Source: CAD feature listing. Evaluate the final solid. Frame: model axes, mm. A direction names the side the tool comes from. Give positions to 0.01 mm unless a question says otherwise; leave off trailing zeros. Loops run counter-clockwise (first coordinate to the right, second up) from the corner with the lowest first, then second, coordinate; pieces in that order, holes last. Notation, with made-up numbers: (57.25, -35) -> (67.25, -35) arc R19 cw to (67.25, -19) -> close; hole circle Ø10 at (-11, 67.25). An arc over 180 degrees is marked (long way). Return JSON: item names as keys, results as strings. Group by question number.
```python
from build123d import *

# Parameters (mm, degrees)
SKETCH1_W           = 24.4
SKETCH1_H           = 14
SKETCH1_R           = 1.3
BOSS_EXTRUDE1_DEPTH = 2.6
SKETCH2_W           = 24.4
SKETCH2_H           = 5
BOSS_EXTRUDE2_DEPTH = 11
SKETCH3_R           = 1.6
CUT_EXTRUDE1_DEPTH  = 4.6


with BuildPart() as part:
    # Sketch1 → Boss-Extrude1 (new body)
    with BuildSketch(Plane.XY):
        with Locations((0, 7)):
            Rectangle(SKETCH1_W, SKETCH1_H)
        with Locations((-8.89, 10.6)):
            Circle(SKETCH1_R, mode=Mode.SUBTRACT)
        with Locations((8.89, 10.6)):
            Circle(SKETCH1_R, mode=Mode.SUBTRACT)
    extrude(amount=BOSS_EXTRUDE1_DEPTH)

    # Sketch2 → Boss-Extrude2 (add)
    with BuildSketch(Plane.XY):
        with Locations((0, 2.5)):
            Rectangle(SKETCH2_W, SKETCH2_H)
    extrude(amount=BOSS_EXTRUDE2_DEPTH)

    # Sketch3 → Cut-Extrude1 (cut)
    with BuildSketch(Plane.XY.offset(11)):
        with Locations((-9.75, 2.2)):
            Circle(SKETCH3_R)
        with Locations((9.75, 2.2)):
            Circle(SKETCH3_R)
    extrude(amount=-CUT_EXTRUDE1_DEPTH, mode=Mode.SUBTRACT)


solid = part.part
```
1) Cut plane D-D on z = 3. Return loops of the section in (x, y), then the cut area to 3 significant figures.
2) Material intervals for line 1 (Y direction, x = -9.75, z = 8.9); line 2 (Z direction, x = 10, y = 8); line 3 (X direction, y = 2, z = 6.5), sorted ascending.
3) Reachability of faces 4 (the face through (0, 7, 0)), 5 (the face through (-10, 2, 6.4)), 6 (the face through (0, 10, 2.6)) from +Z, -Z, +X, -X, +Y, -Y: full face, straight path, thin tool, end or side. Return the list, or none.
4) Cut plane B-B on x = -8.75. Return loops of the section in (y, z), then the cut area to 3 significant figures.
5) Cut plane C-C on y = 10.6. Return loops of the section in (x, z).
6) Cut plane A-A on z = 1.5. Return loops of the section in (x, y), then the cut area to 3 significant figures.
7) Mould query, pull axis Y, two halves, no side actions, for faces 1 (the face through (0, 5, 7)), 2 (the face through (0, 0, 5)), 3 (the face through (8.15, 2.27, 8.73)). Classes: released by +Y, released by -Y, zero draft, split by the parting line, or undercut.
8) Contact query for flat-ended pins moving along their axis: P1, Ø1, axis at x = 9.5, y = 2.5, coming from the +Z side; P2, Ø3.5, axis at x = -8.89, y = 10.6, coming from the +Z side; P3, Ø2, axis at x = -4, z = 10, coming from the +Y side; P4, Ø5, axis at x = -9.75, y = 2.2, coming from the +Z side. Output: stop coordinate, or through.
Calculated:
{
 "1": {"outline": "(-12.2, 0) -> (12.2, 0) -> (12.2, 5) -> (-12.2, 5) -> close", "area": "122 mm2"},
 "2": {"line 1": "0 to 0.6, 3.8 to 5", "line 2": "0 to 2.6", "line 3": "-12.2 to -11.34, -8.16 to 8.16, 11.34 to 12.2"},
 "3": {"face 4": "-Z, +X, -X, +Y, -Y", "face 5": "+Z", "face 6": "+Z, +X, -X, +Y"},
 "4": {"outline": "(0, 0) -> (9.31, 0) -> (9.31, 2.6) -> (5, 2.6) -> (5, 11) -> (3.45, 11) -> (3.45, 6.4) -> (0.95, 6.4) -> (0.95, 11) -> (0, 11) -> close; (11.89, 0) -> (14, 0) -> (14, 2.6) -> (11.89, 2.6) -> close", "area": "60.2 mm2"},
 "5": {"outline": "(-12.2, 0) -> (-10.19, 0) -> (-10.19, 2.6) -> (-12.2, 2.6) -> close; (-7.59, 0) -> (7.59, 0) -> (7.59, 2.6) -> (-7.59, 2.6) -> close; (10.19, 0) -> (12.2, 0) -> (12.2, 2.6) -> (10.19, 2.6) -> close"},
 "6": {"outline": "(-12.2, 0) -> (12.2, 0) -> (12.2, 14) -> (-12.2, 14) -> close; hole circle Ø2.6 at (-8.89, 10.6); hole circle Ø2.6 at (8.89, 10.6)", "area": "331 mm2"},
 "7": {"face 1": "released by +Y", "face 2": "released by -Y", "face 3": "undercut"},
 "8": {"P1": "z = 6.4", "P2": "z = 2.6", "P3": "y = 5", "P4": "z = 11"}
}
